```python
from build123d import *

# Parameters (mm, degrees)
SKETCH1_W           = 120
SKETCH1_H           = 72
SKETCH1_R           = 4.95970326
BOSS_EXTRUDE1_DEPTH = 10
FILLET1_R           = 12
CUT_EXTRUDE1_DEPTH  = 73
SKETCH3_W           = 50
SKETCH3_H           = 72
BOSS_EXTRUDE2_DEPTH = 3


with BuildPart() as part:
    # Sketch1 → Boss-Extrude1 (new body)
    with BuildSketch(Plane(origin=(0, 0, 0), x_dir=(1, 0, 0), z_dir=(0, 1, 0))):
        Rectangle(SKETCH1_W, SKETCH1_H)
        with Locations(Location((-48, 24, 0), (0, 0, 270))):
            Circle(SKETCH1_R, mode=Mode.SUBTRACT)
        with Locations(Location((48, 24, 0), (0, 0, 90))):
            Circle(SKETCH1_R, mode=Mode.SUBTRACT)
        with Locations(Location((48, -24, 0), (0, 0, 270))):
            Circle(SKETCH1_R, mode=Mode.SUBTRACT)
        with Locations(Location((-48, -24, 0), (0, 0, 90))):
            Circle(SKETCH1_R, mode=Mode.SUBTRACT)
    extrude(amount=BOSS_EXTRUDE1_DEPTH)

    # Fillet1
    fillet1_edges = [part.edges().sort_by_distance(p)[0] for p in [
        (60, 5, 36),
        (-60, 5, 36),
        (-60, 5, -36),
        (60, 5, -36),
    ]]
    fillet(fillet1_edges, radius=FILLET1_R)

    # Sketch2 → Cut-Extrude1 (cut)
    with BuildSketch(Plane.XY.offset(36)):
        Polygon((-28, 0), (0, 0), (0, 3), (-25, 3), align=None)
        Polygon((0, 3), (0, 0), (28, 0), (25, 3), align=None)
    extrude(amount=-CUT_EXTRUDE1_DEPTH, mode=Mode.SUBTRACT)

    # Sketch3 → Boss-Extrude2 (add)
    with BuildSketch(Plane(origin=(0, 10, 0), x_dir=(1, 0, 0), z_dir=(0, 1, 0))):
        Rectangle(SKETCH3_W, SKETCH3_H)
    extrude(amount=BOSS_EXTRUDE2_DEPTH)


solid = part.part
```
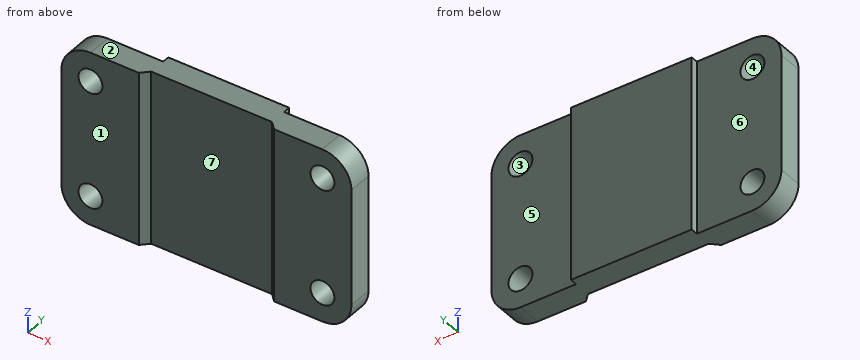
For this review, take the finished solid that the model builds, in its own axes (mm). Face numbers are marked on the shaded views. A direction names the side the tool comes from. Coordinates: 2 decimals unless noted, no trailing zeros. Loops run counter-clockwise (first coordinate to the right, second up) from the corner with the lowest first, then second, coordinate; pieces in that order, holes last. Notation, with made-up numbers: (33.25, -23.75) -> (46.25, -23.75) arc R32 cw to (46.25, 2.25) -> close; hole circle Ø3 at (-9, 34.25). An arc over 180 degrees is marked (long way). Return JSON: item names as keys, results as strings. Group by question number.
(1) Mouldability with a two-part tool opening along Z and no side actions: class the marked faces 1, 2, 3 and 4 as pulls with the +Z half, pulls with the -Z half, needs draft (parallel to the pull), parting line crosses it, or undercut.
(2) Tool access review of the marked faces 5, 6 and 7: name each direction out of +Z, -Z, +X, -X, +Y, -Y from which nothing blocks a thin tool from reaching the whole face with its end or side.
(3) Consider section A-A, the plane x = -46. Give the boundary of the cut face in (y, z).
(4) Consider section D-D, the plane z = 26.5. Give the boundary of the cut face in (x, y), plus the area to 3 significant figures.
(5) For pin 1 Ø5 at (x, z) = (-43.5, -20.5) entering from -Y; pin 2 Ø17.5 at (x, z) = (-48.5, -13) entering from +Y; pin 3 Ø2 at (x, z) = (4, 10.5) entering from -Y; pin 4 Ø1.5 at (y, z) = (11.5, -3.5) entering from -X, all flat-tipped, find the tip position at first contact; note any pin that passes through.
(6) To check wall thickness, follow L1, parallel to X at y = 7, z = 24; L2, parallel to X at y = 2.5, z = 24; L3, parallel to Y at x = 1, z = -17. State the ranges of each line that lie inside material, in increasing order.
(7) Consider section C-C, the plane z = -4.5. Give the boundary of the cut face in (x, y), plus the area to 3 significant figures.
(8) Consider section B-B, the plane y = 7.75. Give the boundary of the cut face in (x, z).
Results below:
{
 "1": {"face 1": "needs draft", "face 2": "pulls with the +Z half", "face 3": "undercut", "face 4": "undercut"},
 "2": {"face 5": "+Z, -Z, +X, +Y", "face 6": "+Z, -Z, -X, +Y", "face 7": "+Z, -Z, -Y"},
 "3": {"outline": "(0, -36) -> (10, -36) -> (10, -28.54) -> (0, -28.54) -> close; (0, -19.46) -> (10, -19.46) -> (10, 19.46) -> (0, 19.46) -> close; (0, 28.54) -> (10, 28.54) -> (10, 36) -> (0, 36) -> close"},
 "4": {"outline": "(-59.74, 0) -> (-52.28, 0) -> (-52.28, 10) -> (-59.74, 10) -> close; (-43.72, 0) -> (-28, 0) -> (-25, 3) -> (25, 3) -> (28, 0) -> (43.72, 0) -> (43.72, 10) -> (25, 10) -> (25, 13) -> (-25, 13) -> (-25, 10) -> (-43.72, 10) -> close; (52.28, 0) -> (59.74, 0) -> (59.74, 10) -> (52.28, 10) -> close", "area": "1,010 mm2"},
 "5": {"pin 1": "stops at y = 0", "pin 2": "stops at y = 10", "pin 3": "stops at y = 3", "pin 4": "stops at x = -25"},
 "6": {"L1": "x = -60 to -52.96, -43.04 to 43.04, 52.96 to 60", "L2": "x = -60 to -52.96, -43.04 to -25.5, 25.5 to 43.04, 52.96 to 60", "L3": "y = 3 to 13"},
 "7": {"outline": "(-60, 0) -> (-28, 0) -> (-25, 3) -> (25, 3) -> (28, 0) -> (60, 0) -> (60, 10) -> (25, 10) -> (25, 13) -> (-25, 13) -> (-25, 10) -> (-60, 10) -> close", "area": "1,190 mm2"},
 "8": {"outline": "(-60, -24) arc R12 ccw to (-48, -36) -> (48, -36) arc R12 ccw to (60, -24) -> (60, 24) arc R12 ccw to (48, 36) -> (-48, 36) arc R12 ccw to (-60, 24) -> close; hole circle Ø9.92 at (-48, -24); hole circle Ø9.92 at (-48, 24); hole circle Ø9.92 at (48, -24); hole circle Ø9.92 at (48, 24)"}
}
